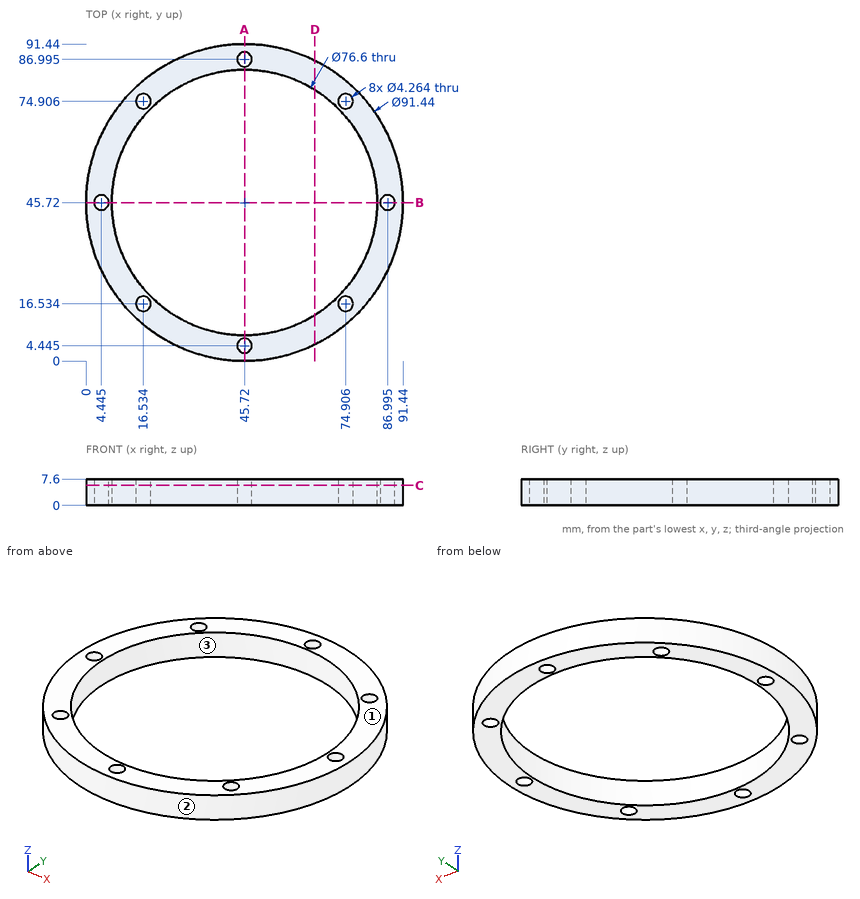
Geometry: see drawing. Coordinates: mm, zero at the bounding-box minimum. Round coordinates to 2 decimals unless told otherwise and drop trailing zeros. Order: outer loops, then holes, each group sorted by start corner. A loop starts at its lowest first (then second) coordinate and runs counter-clockwise, first axis right, second up. Notation, with made-up numbers: (52, -35) - (103, -35) arc R26 cw to (103, -11) - close; hole circle Ø6 at (42, -19.75). An arc over 180 degrees is marked (long way). One line per question, with ' | ' between items. Start each with the question number.
1) Cut plane C-C, the plane z = 5.75. Give the number of separate pieces and of enclosed holes in the cut face, then the cut area to 3 significant figures.
2) Cut plane A-A, the plane x = 45.72. Return the cut outline in (y, z).
3) Pull-direction query (X, two-part tool) for the marked faces 1, 2 and 3; classes: +X half, -X half, draft (parallel to the pull), parting line (faces both ways), or undercut.
4) Contact query for flat-ended pins moving along their axis: P1, Ø3, axis at y = 14.5, z = 3, coming from the -X side; P2, Ø4, axis at y = 23.5, z = 4, coming from the -X side; P3, Ø4, axis at y = 34.5, z = 1.5, coming from the +X side. Output: stop coordinate, or through.
5) Cut plane D-D, the plane x = 66. Return the cut outline in (y, z), then the cut area to 3 significant figures.
6) Ray query, probe 1 along X at (y, z) = (53.5, 4); probe 2 along Y at (x, z) = (13.5, 4.75) (1 decimal); probe 3 along X at (y, z) = (14, 4.75) (1 decimal). Return the intervals inside material, ascending.
Worked out:
1) separate pieces: 1 | enclosed holes: 9 | area: 1,840 mm^2
2) outline: (0, 0) - (2.31, 0) - (2.31, 7.6) - (0, 7.6) - close; (6.58, 0) - (7.42, 0) - (7.42, 7.6) - (6.58, 7.6) - close; (84.02, 0) - (84.86, 0) - (84.86, 7.6) - (84.02, 7.6) - close; (89.13, 0) - (91.44, 0) - (91.44, 7.6) - (89.13, 7.6) - close
3) face 1: draft | face 2: parting line | face 3: undercut
4) P1: stops at x = 10.98 | P2: stops at x = 4.71 | P3: stops at x = 90.5
5) outline: (4.74, 0) - (13.23, 0) - (13.23, 7.6) - (4.74, 7.6) - close; (78.21, 0) - (86.7, 0) - (86.7, 7.6) - (78.21, 7.6) - close | area: 129 mm^2
6) probe 1: x = 0.67 to 8.22, 83.22 to 90.77 | probe 2: y = 13.3 to 25, 66.4 to 78.2 | probe 3: x = 12.8 to 24.3, 67.2 to 78.6
